Build history of the part. All positions in model axes, mm. Coordinates: 2 decimals unless noted, no trailing zeros. Order: outer loops, then holes, each group sorted by start corner. A loop starts at its lowest first (then second) coordinate and runs counter-clockwise, first axis right, second up. Notation, with made-up numbers: (-29.5, -30) - (-23.5, -30) arc R19 ccw to (-23.5, -8) - close; hole circle Ø2 at (-17.75, 72.25). An arc over 180 degrees is marked (long way). One line per item, written item: value.
from build123d import *

# Parameters (mm, degrees)
SKETCH1_W           = 609.6
SKETCH1_H           = 342.9
SKETCH1_R           = 2.555
SKETCH1_W_2         = 500
SKETCH1_H_2         = 150
BOSS_EXTRUDE1_DEPTH = 6.35


with BuildPart() as part:
    # Sketch1 → Boss-Extrude1 (new body)
    with BuildSketch(Plane(origin=(0, 0, 0), x_dir=(1, 0, 0), z_dir=(0, 1, 0))):
        with Locations((304.8, 171.45)):
            Rectangle(SKETCH1_W, SKETCH1_H)
        with Locations((404.8, 256.45)):
            Circle(SKETCH1_R, mode=Mode.SUBTRACT)
        with Locations((404.8, 86.45)):
            Circle(SKETCH1_R, mode=Mode.SUBTRACT)
        with Locations((304.8, 171.45)):
            Rectangle(SKETCH1_W_2, SKETCH1_H_2, mode=Mode.SUBTRACT)
    extrude(amount=BOSS_EXTRUDE1_DEPTH)


solid = part.part
1. Flat gauge pins, fed straight in: P1, Ø3, axis at y = 2, z = -106.5, coming from the -X side; P2, Ø3, axis at x = 404.8, z = -86.45, coming from the +Y side. Where does each tip first touch, or does it go through?
Values found:
P1: stops at x = 0
P2: passes through
2. Band-saw the part on B-B, the plane z = -115. Give the cut face in (x, y), and give its area (3 significant figures).
Values found:
outline: (0, 0) - (54.8, 0) - (54.8, 6.35) - (0, 6.35) - close; (554.8, 0) - (609.6, 0) - (609.6, 6.35) - (554.8, 6.35) - close
area: 696 mm2
3. Band-saw the part on C-C, the plane y = 2. Give the cut face in (x, z) (3 decimals).
Values found:
outline: (0, -342.9) - (609.6, -342.9) - (609.6, 0) - (0, 0) - close; hole (54.8, -246.45) - (554.8, -246.45) - (554.8, -96.45) - (54.8, -96.45) - close; hole circle Ø5.11 at (404.8, -256.45); hole circle Ø5.11 at (404.8, -86.45)
4. Probe line 1 along Z through (x, y) = (404.8, 4) (3 decimals); line 2 along X through (y, z) = (4.75, -86.45) (3 decimals); line 3 along X through (y, z) = (3.5, -175). List the from-to ranges inside material, lowest first.
Values found:
line 1: z = -342.9 to -259.005, -253.895 to -246.45, -96.45 to -89.005, -83.895 to 0
line 2: x = 0 to 402.245, 407.355 to 609.6
line 3: x = 0 to 54.8, 554.8 to 609.6
5. Band-saw the part on A-A, the plane x = 341. Give the cut face in (y, z).
Values found:
outline: (0, -342.9) - (6.35, -342.9) - (6.35, -246.45) - (0, -246.45) - close; (0, -96.45) - (6.35, -96.45) - (6.35, 0) - (0, 0) - close
